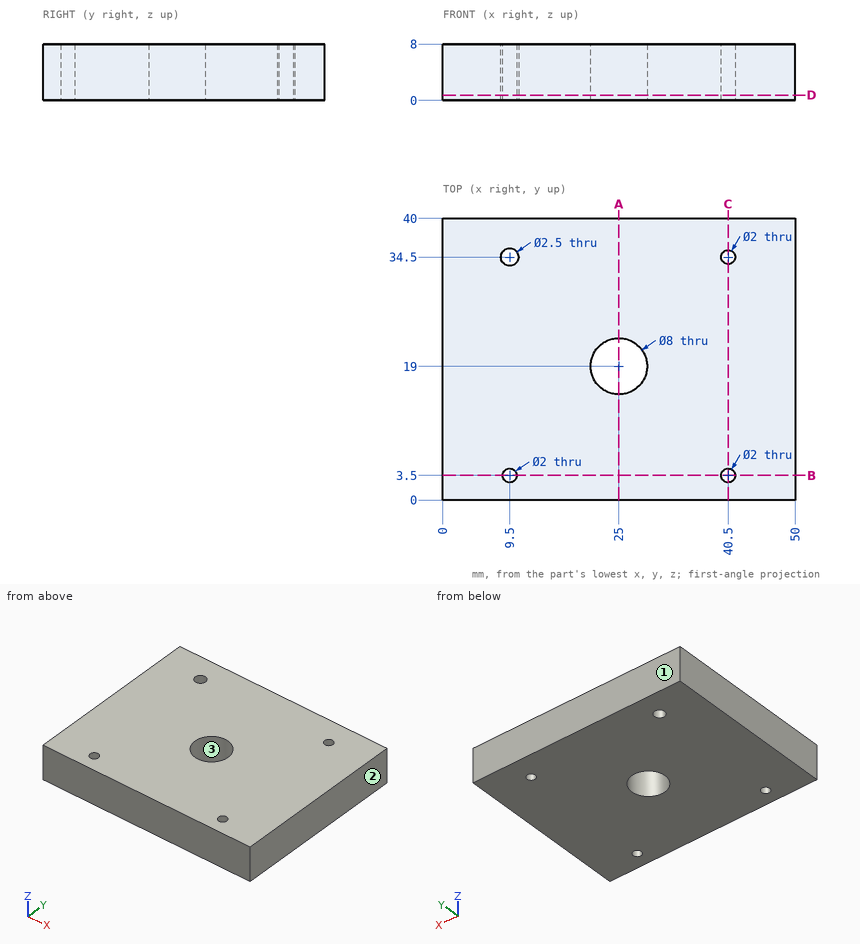
Can you work these out from the drawing? Everything is in mm from the part's minimum corner. Round coordinates to 2 decimals unless told otherwise and drop trailing zeros. Loops run counter-clockwise (first coordinate to the right, second up) from the corner with the lowest first, then second, coordinate; pieces in that order, holes last. Notation, with made-up numbers: M -12.5,-21.5 L 38.5,-21.5 A16 cw 38.5,6.5 Z; hole C 48,56 d8. An arc over 180 degrees is marked long. Answer in a Markdown table with one row per item.
1. If we section it at B-B, the plane y = 3.5: Please give me the cut outline in (x, z).
Established:
| item | result |
|---|---|
| outline | M 0,0 L 8.5,0 L 8.5,8 L 0,8 Z; M 10.5,0 L 39.5,0 L 39.5,8 L 10.5,8 Z; M 41.5,0 L 50,0 L 50,8 L 41.5,8 Z |
2. Please list where these lines run through material, in increasing order: line 1 (Y direction, x = 40.5, z = 3); line 2 (Y direction, x = 9.5, z = 4.75); line 3 (Y direction, x = 25, z = 4.5). Write a range as from..to.
Established:
| item | result |
|---|---|
| line 1 | 0..2.5, 4.5..33.5, 35.5..40 |
| line 2 | 0..2.5, 4.5..33.25, 35.75..40 |
| line 3 | 0..15, 23..40 |
3. Thinking about a two-plate mould opening in Y: for the marked faces 1, 2 and 3, which applies, pulls with the +Y half, pulls with the -Y half, needs draft (parallel to the pull), parting line crosses it, or undercut?
Established:
| item | result |
|---|---|
| face 1 | pulls with the +Y half |
| face 2 | needs draft |
| face 3 | undercut |
4. If we section it at C-C, the plane x = 40.5: Please give me the cut outline in (y, z), plus the area to 3 significant figures.
Established:
| item | result |
|---|---|
| outline | M 0,0 L 2.5,0 L 2.5,8 L 0,8 Z; M 4.5,0 L 33.5,0 L 33.5,8 L 4.5,8 Z; M 35.5,0 L 40,0 L 40,8 L 35.5,8 Z |
| area | 288 mm² |
5. If we section it at A-A, the plane x = 25: Please give me the cut outline in (y, z).
Established:
| item | result |
|---|---|
| outline | M 0,0 L 15,0 L 15,8 L 0,8 Z; M 23,0 L 40,0 L 40,8 L 23,8 Z |
6. If we section it at D-D, the plane z = 0.75: Please give me the cut outline in (x, y).
Established:
| item | result |
|---|---|
| outline | M 0,0 L 50,0 L 50,40 L 0,40 Z; hole C 9.5,34.5 d2.5; hole C 9.5,3.5 d2; hole C 25,19 d8; hole C 40.5,3.5 d2; hole C 40.5,34.5 d2 |
